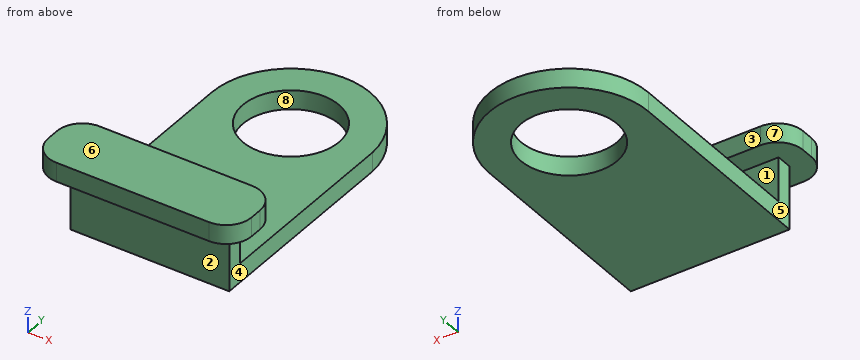
```python
from build123d import *

# Parameters (mm, degrees)
F0_R     = 7.5625599735
F0_W     = 25
F0_H     = 3.598708484
F0_H_2   = 2.5
F1_DEPTH = 3
F2_DEPTH = 10
F3_START = 10
F3_DEPTH = 3
F4_R     = 4


with BuildPart() as f1:
    # F0 (on Top) → F1 (new body)
    with BuildSketch(Plane.XY):
        with BuildLine():
            Line((-11.908370629, 31.2152840197), (-11.908370629, 4.7718174662))
            Line((-11.908370629, 4.7718174662), (13.091629371, 4.7718174662))
            Line((13.091629371, 4.7718174662), (13.091629371, 31.7831486464))
            ThreePointArc((13.091629371, 31.7831486464), (0.3140732241, 43.7185083062), (-11.908370629, 31.2152840197))
        make_face()
        with Locations((0.5980787757, 31.2152840197)):
            Circle(F0_R, mode=Mode.SUBTRACT)
        with Locations((0.591629371, 2.9724632242)):
            Rectangle(F0_W, F0_H)
        with Locations((0.591629371, -0.0768910178)):
            Rectangle(F0_W, F0_H_2)
    extrude(amount=F1_DEPTH)

    # F0 (on Top) → F2 (join)
    with BuildSketch(Plane.XY):
        with Locations((0.591629371, -0.0768910178)):
            Rectangle(F0_W, F0_H_2)
    extrude(amount=F2_DEPTH)

    # F0 (on Top) → F3 (join)
    with BuildSketch(Plane.XY.offset(F3_START)):
        with Locations((0.591629371, 2.9724632242)):
            Rectangle(F0_W, F0_H)
        Polygon((-11.908370629, -1.3268910178), (-11.908370629, 1.1731089822), (-11.908370629, 4.7718174662), (-15.4697376937, 4.7718174662), (-15.4697376937, -5.2281825338), (16.5302623063, -5.2281825338), (16.5302623063, 4.7718174662), (13.091629371, 4.7718174662), (13.091629371, 1.1731089822), (13.091629371, -1.3268910178), align=None)
        with Locations((0.591629371, -0.0768910178)):
            Rectangle(F0_W, F0_H_2)
    extrude(amount=F3_DEPTH)

    # F4
    f4_edges = [f1.edges().sort_by_distance(p)[0] for p in [
        (16.530262, -5.228183, 11.5),
        (16.530262, 4.771817, 11.5),
        (-15.469738, -5.228183, 11.5),
        (-15.469738, 4.771817, 11.5),
    ]]
    fillet(f4_edges, radius=F4_R)


solid = f1.part
```
Verification items for the finished model (mm, model axes). Face numbers are marked on the shaded views. A direction names the side the tool comes from. Coordinates: 2 decimals unless noted, no trailing zeros. Write each loop counter-clockwise with the first axis right and the second up, starting at its lowest first coordinate (ties: lowest second). Pieces come first, ordered by that corner, then holes. Notation, with made-up numbers: (-16, 73.5) - (19, 73.5) arc R7 cw to (19, 84.5) - close; hole circle Ø3 at (82, 5.25). An arc over 180 degrees is marked (long way). Write item = value, one per line.
Q1. Cross-section at C-C (z = 2.5). Enter the section's corners in (x, y).
Answer:
outline = (-11.91, -1.33) - (13.09, -1.33) - (13.09, 31.78) arc R12.51 ccw to (-11.91, 31.22) - close; hole circle Ø15.13 at (0.6, 31.22)
Q2. Go/stop test with flat-tipped pins: pin 1 Ø2 at (x, y) = (-4, 37) entering from +Z; pin 2 Ø5 at (x, z) = (-3, 7) entering from -Y; pin 3 Ø1 at (x, z) = (12, 8) entering from +Y. Record where each tip stops, or that it passes through.
Answer:
pin_1 = 3
pin_2 = -1.33
pin_3 = 1.17
Q3. Access from +Z, -Z, +X, -X, +Y, -Y to the whole of each face (thin tool, end or side, straight path). Record for the marked faces 1, 2, 3, 4 and 5.
Answer:
face_1 = +X, -X, +Y
face_2 = -Z, +X, -X, -Y
face_3 = +Z, +X, -X, +Y
face_4 = -Z, +X, +Y, -Y
face_5 = -Z, -X, +Y, -Y
Q4. Cross-section at B-B (y = 35). Enter the section's corners in (x, z), plus the area to 3 significant figures.
Answer:
outline = (-11.32, 0) - (-5.95, 0) - (-5.95, 3) - (-11.32, 3) - close; (7.15, 0) - (12.52, 0) - (12.52, 3) - (7.15, 3) - close
area = 32.2 mm²
Q5. Cross-section at D-D (x = -9). Enter the section's corners in (y, z), plus the area to 3 significant figures.
Answer:
outline = (-5.23, 10) - (-1.33, 10) - (-1.33, 0) - (39.23, 0) - (39.23, 3) - (1.17, 3) - (1.17, 10) - (4.77, 10) - (4.77, 13) - (-5.23, 13) - close
area = 169 mm²
Q6. Material ranges on L1, parallel to Z at x = 10, y = 4; L2, parallel to Z at x = 3, y = 14; L3, parallel to Y at x = 12, z = 9, recorded low to high. Write a range as from..to.
Answer:
L1 = 0..3, 10..13
L2 = 0..3
L3 = -1.33..1.17
Q7. Mould release check, pull along X, two halves, no side actions. Record for the marked faces 6, 7 and 8: released by +X, released by -X, zero draft, split by the parting line, or undercut.
Answer:
face_6 = zero draft
face_7 = released by -X
face_8 = undercut
Q8. Cross-section at A-A (x = -4.5). Enter the section's corners in (y, z), plus the area to 3 significant figures.
Answer:
outline = (-5.23, 10) - (-1.33, 10) - (-1.33, 0) - (25.63, 0) - (25.63, 3) - (1.17, 3) - (1.17, 10) - (4.77, 10) - (4.77, 13) - (-5.23, 13) - close; (36.8, 0) - (42.64, 0) - (42.64, 3) - (36.8, 3) - close
area = 146 mm²
